from build123d import *

# Parameters (mm, degrees)
ESQUISSE1_R                  = 22.5
BOSS_EXTRU_1_DEPTH           = 37
ENL_V_MAT_EXTRU_1_DEPTH      = 3
ENL_V_MAT_EXTRU_1_DEPTH_BACK = 34
ESQUISSE4_R                  = 19
ENL_V_MAT_EXTRU_3_DEPTH      = 49.80061475
ESQUISSE9_R                  = 37.5
BOSS_EXTRU_2_DEPTH           = 3
ENL_V_START                  = 3
ESQUISSE4_2_R                = 19
ENL_V_MAT_EXTRU_4_DEPTH      = 3
D_GAGEMENT_M61_D             = 6.4
ENL_V_START_2                = -3
ENL_V_MAT_EXTRU_5_DEPTH      = 3
CONG_1_R                     = 10
CONG_1_OF_SYM_TRIE4_R        = 10
SYM_TRIE5_START              = -3
SYM_TRIE5_DEPTH              = 3


# Read off the part's stored shape, not the designer's step: Symétrie5
with BuildPart() as part:
    # Esquisse1 → Boss.-Extru.1 (new body)
    with BuildSketch(Plane.XY):
        Circle(ESQUISSE1_R)
    extrude(amount=BOSS_EXTRU_1_DEPTH)

    # Esquisse4 → Enlèv. mat.-Extru.1 (cut, two sides: drawn at the far end of the back side and taken through both)
    with BuildSketch(Plane(origin=(0, 0, 0), x_dir=(-1, 0, 0), z_dir=(0, 0, -1)).offset(-ENL_V_MAT_EXTRU_1_DEPTH_BACK)):
        with Locations(Location((0, 0, 0), (0, 0, 180))):
            Circle(ESQUISSE4_R)
    extrude(amount=ENL_V_MAT_EXTRU_1_DEPTH + ENL_V_MAT_EXTRU_1_DEPTH_BACK, mode=Mode.SUBTRACT)

    # Esquisse7 → Enlèv. mat.-Extru.3 (cut, through all)
    with BuildSketch(Plane(origin=(0, 0, 0), x_dir=(-1, 0, 0), z_dir=(0, 0, -1))):
        with BuildLine():
            Line((-14.573529274, -17.142410697), (-11.999578126, -14.731263517))
            ThreePointArc((-11.999578126, -14.731263517), (-17.160885531, -8.154998946), (-19, 0))
            Line((-19, 0), (-22.5, 0))
            ThreePointArc((-22.5, 0), (-20.422468125, -9.443134843), (-14.573529274, -17.142410697))
        make_face()
    extrude(amount=-ENL_V_MAT_EXTRU_3_DEPTH, mode=Mode.SUBTRACT)

    # Esquisse9 → Boss.-Extru.2 (add)
    with BuildSketch(Plane(origin=(0, 0, 0), x_dir=(-1, 0, 0), z_dir=(0, 0, -1))):
        Circle(ESQUISSE9_R)
    extrude(amount=BOSS_EXTRU_2_DEPTH)

    # Esquisse4<2> → Enlèv. mat.-Extru.4 (cut)
    with BuildSketch(Plane(origin=(0, 0, 0), x_dir=(-1, 0, 0), z_dir=(0, 0, -1)).offset(ENL_V_START)):
        with Locations(Location((0, 0, 0), (0, 0, 180))):
            Circle(ESQUISSE4_2_R)
    extrude(amount=-ENL_V_MAT_EXTRU_4_DEPTH, mode=Mode.SUBTRACT)

    # Dégagement M61 (through all)
    with Locations(Plane(origin=(0, 0, -3), x_dir=(-1, 0, 0), z_dir=(0, 0, -1))):
        with Locations((0, 27.5), (27.5, 0), (0, -27.5), (-27.5, 0)):
            Hole(D_GAGEMENT_M61_D / 2)

    # Esquisse15 → Enlèv. mat.-Extru.5 (cut)
    with BuildSketch(Plane(origin=(0, 0, -3), x_dir=(-1, 0, 0), z_dir=(0, 0, -1)).offset(ENL_V_START_2)):
        with BuildLine():
            Line((34.932786702, 13.636363636), (25.617376915, 10))
            ThreePointArc((25.617376915, 10), (19.384796538, 19.505887911), (9.840281362, 25.679152297))
            Line((9.840281362, 25.679152297), (12.051640076, 35.51067405))
            ThreePointArc((12.051640076, 35.51067405), (25.913422274, 27.106171734), (34.932786702, 13.636363636))
        make_face()
    enl_v_mat_extru_5 = extrude(amount=ENL_V_MAT_EXTRU_5_DEPTH, mode=Mode.SUBTRACT)

    # Congé1
    # the kernel refuses this fillet: 10 mm, written as the material it takes off along each edge
    with BuildSketch(Plane(origin=(-12.051640076, 35.51067405, 30.511737931), x_dir=(0.9866266204606564, 0.16299666192405335, 0), z_dir=(0, 0, -1))) as cong_1_piece_1:
        with BuildLine():
            CenterArc((10.577402483, 9.866707582), CONG_1_R, 178.889666711, 100.475681696)
            Line((0.579280147, 10.060485169), (0.3793177, 10.064360721))
            ThreePointArc((0.3793177, 10.064360721), (0.089970794, 5.04173949), (-0.199669279, 0.011496906))
            Line((-0.199669279, 0.011496906), (-0.032545854, -0.197334152))
            ThreePointArc((-0.032545854, -0.197334152), (6.102347586, -0.699846569), (12.237241026, -0.197334152))
            Line((12.237241026, -0.197334152), (12.204695172, 0))
        make_face()
    extrude(amount=64.023475862, mode=Mode.SUBTRACT)
    with BuildSketch(Plane(origin=(-34.932786702, 13.636363636, 34.090909091), x_dir=(-0.18820424606330075, -0.9821299108385533, 0), z_dir=(0, 0, -1))) as cong_1_piece_2:
        with BuildLine():
            CenterArc((11.818181818, -9.83332166), CONG_1_R, 79.524318304, 100.475681696)
            Line((1.818181818, -9.83332166), (1.618181818, -9.83332166))
            ThreePointArc((1.618181818, -9.83332166), (0.712424476, -4.953024467), (-0.196666433, -0.036363636))
            Line((-0.196666433, -0.036363636), (-0.036363636, 0.196666433))
            ThreePointArc((-0.036363636, 0.196666433), (6.818181818, 0.825043774), (13.672727273, 0.196666433))
            Line((13.672727273, 0.196666433), (13.636363636, 0))
        make_face()
    extrude(amount=71.181818182, mode=Mode.SUBTRACT)

    # Symétrie4: Enlèv. mat.-Extru.5 across plane
    add(enl_v_mat_extru_5.mirror(Plane(origin=(0, 0, 0), x_dir=(0, 0, 1), z_dir=(1, 0, 0))), mode=Mode.SUBTRACT)

    # Congé1 of Symétrie4
    # the kernel refuses this fillet: 10 mm, written as the material it takes off along each edge
    with BuildSketch(Plane(origin=(12.051640076, 35.51067405, 30.511737931), x_dir=(-0.9866266204606562, 0.1629966619240532, 0), z_dir=(0, 0, -1))) as cong_1_of_sym_trie4_piece_1:
        with BuildLine():
            CenterArc((10.577402483, -9.866707582), CONG_1_OF_SYM_TRIE4_R, 80.634651593, 100.475681696)
            Line((0.579280147, -10.060485169), (0.3793177, -10.064360721))
            ThreePointArc((0.3793177, -10.064360721), (0.089970794, -5.04173949), (-0.199669279, -0.011496906))
            Line((-0.199669279, -0.011496906), (-0.032545854, 0.197334152))
            ThreePointArc((-0.032545854, 0.197334152), (6.102347586, 0.699846569), (12.237241026, 0.197334152))
            Line((12.237241026, 0.197334152), (12.204695172, 0))
        make_face()
    extrude(amount=64.023475862, mode=Mode.SUBTRACT)
    with BuildSketch(Plane(origin=(34.932786702, 13.636363636, 34.090909091), x_dir=(0.18820424606330144, -0.982129910838553, 0), z_dir=(0, 0, -1))) as cong_1_of_sym_trie4_piece_2:
        with BuildLine():
            CenterArc((11.818181818, 9.83332166), CONG_1_OF_SYM_TRIE4_R, 180, 100.475681696)
            Line((1.818181818, 9.83332166), (1.618181818, 9.83332166))
            ThreePointArc((1.618181818, 9.83332166), (0.712424476, 4.953024467), (-0.196666433, 0.036363636))
            Line((-0.196666433, 0.036363636), (-0.036363636, -0.196666433))
            ThreePointArc((-0.036363636, -0.196666433), (6.818181818, -0.825043774), (13.672727273, -0.196666433))
            Line((13.672727273, -0.196666433), (13.636363636, 0))
        make_face()
    extrude(amount=71.181818182, mode=Mode.SUBTRACT)

    # Symétrie5 outline → Symétrie5 (cut)
    with BuildSketch(Plane.XY.offset(SYM_TRIE5_START)):
        with BuildLine():
            ThreePointArc((-0.010162924, -37.499998623), (-7.696247071, -33.893936965), (-9.840281362, -25.679152297))
            ThreePointArc((-9.840281362, -25.679152297), (-19.384796538, -19.505887911), (-25.617376915, -10))
            ThreePointArc((-25.617376915, -10), (-33.845353653, -7.907162456), (-37.499208239, -0.243683034))
            ThreePointArc((-37.499208239, -0.243683034), (-26.433813461, -26.59893806), (-0.010162924, -37.499998623))
        make_face()
        with BuildLine():
            ThreePointArc((9.840281362, -25.679152297), (7.696247071, -33.893936965), (0.010162924, -37.499998623))
            ThreePointArc((0.010162924, -37.499998623), (26.433813461, -26.59893806), (37.499208239, -0.243683034))
            ThreePointArc((37.499208239, -0.243683034), (33.845353653, -7.907162456), (25.617376915, -10))
            ThreePointArc((25.617376915, -10), (19.384796538, -19.505887911), (9.840281362, -25.679152297))
        make_face()
    extrude(amount=SYM_TRIE5_DEPTH, mode=Mode.SUBTRACT)


solid = part.part
Geometry check sheet. Reference: the model listing, model coordinates, mm. A direction names the side the tool comes from. Round coordinates to 2 decimals unless told otherwise and drop trailing zeros. Loops run counter-clockwise (first coordinate to the right, second up) from the corner with the lowest first, then second, coordinate; pieces in that order, holes last. Notation, with made-up numbers: (34, -33) -> (74, -33) arc R18 ccw to (74, 2) -> close; hole circle Ø10 at (-29.75, 31.25). An arc over 180 degrees is marked (long way). Answer as a JSON object with one key per item and string values. Group by question number.
Item 1: Cross-section at A-A, the plane y = -27.5. Record the cut outline in (x, z).
Item 2: Thickness scan on line 1 along Y through (x, z) = (0, -1.95); line 2 along Y through (x, z) = (0, 18); line 3 along Z through (x, y) = (-11, 11). Record the ranges inside material, lowest first.
Item 3: Depth check by flat-ended pin: pin 1 Ø1 at (x, z) = (21, 13) entering from -Y; pin 2 Ø4 at (x, z) = (0, 17.5) entering from +Y; pin 3 Ø4 at (x, y) = (27, -7) entering from +Z. Enter the tip coordinate at first touch or a pass-through.
Item 4: Set-up check for faces 1 (the face through (21, 0, 18)), 2 (the face through (-20.05, 10.21, 18.24)), 3 (the face through (13.3, -15.95, 18.24)), 4 (the face through (0, 20, -3)): record each of +Z, -Z, +X, -X, +Y, -Y from which the full face is reachable in a straight line by a thin tool's end or side.
Item 5: Cross-section at B-B, the plane x = 27.5. Record the cut outline in (y, z), plus the area to 3 significant figures.
Item 6: Cross-section at D-D, the plane y = 8. Record the cut outline in (x, z).
Item 7: Cross-section at C-C, the plane z = 29. Record the cut outline in (x, y), plus the area to 3 significant figures.
Item 8: Release check for a two-part mould opening along X. For faces 5 (the face through (-7.774, 33.799, -1.479)), 6 (the face through (20, -3, 0)), 7 (the face through (-0.417, -24.327, -1.479)) record: pulls with the +X half, pulls with the -X half, needs draft (parallel to the pull), parting line crosses it, or undercut.
Determined:
{
 "1": {"outline": "(-10.01, -3) -> (-3.2, -3) -> (-3.2, 0) -> (-10.01, 0) -> close; (3.2, -3) -> (10.01, -3) -> (10.01, 0) -> (3.2, 0) -> close"},
 "2": {"line 1": "y = -37.5 to -30.7, -24.3 to -19, 19 to 24.3, 30.7 to 37.5", "line 2": "y = -22.5 to -19, 19 to 22.5", "line 3": "z = 34 to 37"},
 "3": {"pin 1": "stops at y = 0", "pin 2": "stops at y = 22.5", "pin 3": "stops at z = 0"},
 "4": {"face 1": "+Z, +X, -Y", "face 2": "+Z", "face 3": "+Z, +X", "face 4": "-Z, +X, -X, +Y, -Y"},
 "5": {"outline": "(-10.18, -3) -> (-3.2, -3) -> (-3.2, 0) -> (-10.18, 0) -> close; (3.2, -3) -> (10.18, -3) -> (10.18, 0) -> (3.2, 0) -> close", "area": "41.9 mm²"},
 "6": {"outline": "(-33.73, -3) -> (-17.23, -3) -> (-17.23, 34) -> (17.23, 34) -> (17.23, -3) -> (33.73, -3) -> (33.73, 0) -> (21.03, 0) -> (21.03, 37) -> (-21.03, 37) -> (-21.03, 0) -> (-33.73, 0) -> close"},
 "7": {"outline": "(12, -14.73) arc R19 cw (long way) to (19, 0) -> (22.5, 0) arc R22.5 ccw (long way) to (14.57, -17.14) -> close", "area": "393 mm²"},
 "8": {"face 5": "pulls with the -X half", "face 6": "needs draft", "face 7": "undercut"}
}
